from build123d import *

# Parameters (mm, degrees)
F0_R     = 2.5
F1_DEPTH = 6


with BuildPart() as f1:
    # F0 (on Top) → F1 (new body)
    with BuildSketch(Plane.XY):
        with BuildLine():
            ThreePointArc((4.796656, 79.382457), (0.466529, 81.882457), (-3.863598, 79.382457))
            Line((-3.863598, 79.382457), (-70.203344, -35.521353))
            ThreePointArc((-70.203344, -35.521353), (-70.203344, -40.521353), (-65.873217, -43.021353))
            Line((-65.873217, -43.021353), (66.806275, -43.021353))
            ThreePointArc((66.806275, -43.021353), (71.136402, -40.521353), (71.136402, -35.521353))
            Line((71.136402, -35.521353), (4.796656, 79.382457))
        make_face()
        with Locations((-65.873217, -38.021353)):
            Circle(F0_R, mode=Mode.SUBTRACT)
        with Locations((66.806275, -38.021353)):
            Circle(F0_R, mode=Mode.SUBTRACT)
        with Locations((0.466529, 76.882457)):
            Circle(F0_R, mode=Mode.SUBTRACT)
    extrude(amount=F1_DEPTH)


solid = f1.part
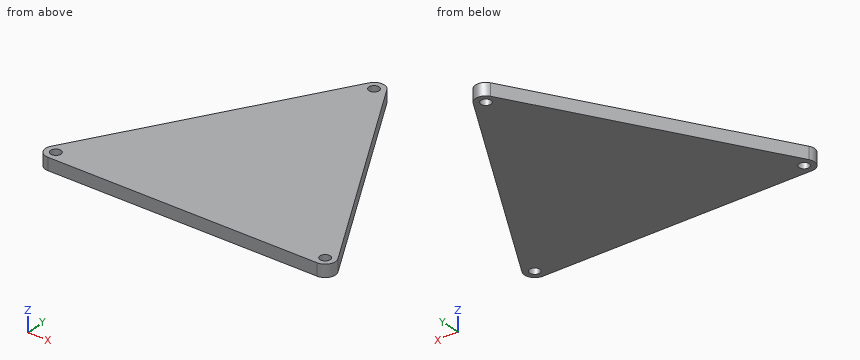
Model file for the job. Use its own axes, mm. Coordinates: 2 decimals unless noted, no trailing zeros. Order: outer loops, then holes, each group sorted by start corner. A loop starts at its lowest first (then second) coordinate and runs counter-clockwise, first axis right, second up. Notation, with made-up numbers: M 40,65 L 52,65 A33 ccw 52,93 Z; hole C -38,50.25 d1. An arc over 180 degrees is marked long. Return JSON: item names as keys, results as strings.
1. Saw through at A-A (z = 3.65). Give the cut face in (x, y).
Ans:
{"outline": "M -70.2,-35.52 A5 ccw -65.87,-43.02 L 66.81,-43.02 A5 ccw 71.14,-35.52 L 4.8,79.38 A5 ccw -3.86,79.38 Z; hole C -65.87,-38.02 d5; hole C 0.47,76.88 d5; hole C 66.81,-38.02 d5"}
2. Saw through at B-B (x = 17). Give the cut face in (y, z), and give its area (3 significant figures).
Ans:
{"outline": "M -43.02,0 L 58.25,0 L 58.25,6 L -43.02,6 Z", "area": "608 mm^2"}
3. Drill centre lines: probe 1 along Y at (x, z) = (66, 3.45); probe 2 along Y at (x, z) = (60, 0.9); probe 3 along Y at (x, z) = (7, 1.05). Where is each one in solid material? Low to high.
Ans:
{"probe 1": "-43.02 to -40.39, -35.65 to -26.62", "probe 2": "-43.02 to -16.23", "probe 3": "-43.02 to 75.57"}
4. Flat gauge pins, fed straight in: pin 1 (3 mm diameter, centred on x = -65.87, y = -38.02, fed in from +Z); pin 2 (1 mm diameter, centred on y = 35.5, z = 2, fed in from -X). Where does each tip first touch, or does it go through?
Ans:
{"pin 1": "through", "pin 2": "x = -29.49"}
5. Saw through at C-C (y = 9). Give the cut face in (x, z), and give its area (3 significant figures).
Ans:
{"outline": "M -44.5,0 L 45.43,0 L 45.43,6 L -44.5,6 Z", "area": "540 mm^2"}
